```python
from build123d import *

# Parameters (mm, degrees)
SKETCH1_R           = 4
BOSS_EXTRUDE1_DEPTH = 4
SKETCH4_R           = 7
BOSS_EXTRUDE2_DEPTH = 5
SKETCH2_R           = 4.5
SKETCH3_R           = 4


with BuildPart() as part:
    # Sketch1 → Boss-Extrude1 (new body)
    with BuildSketch(Plane(origin=(0, 0, 0), x_dir=(1, 0, 0), z_dir=(0, 1, 0))):
        with BuildLine():
            Line((-3, 300), (-3, 6.32455532))
            ThreePointArc((-3, 6.32455532), (0, -7), (3, 6.32455532))
            Line((3, 6.32455532), (3, 300))
            Line((3, 300), (4.701562119, 301.701562119))
            ThreePointArc((4.701562119, 301.701562119), (4.924825408, 300.863767737), (5, 300))
            Line((5, 300), (10, 300))
            ThreePointArc((10, 300), (0, 310), (-10, 300))
            Line((-10, 300), (-5, 300))
            ThreePointArc((-5, 300), (-4.924825408, 300.863767737), (-4.701562119, 301.701562119))
            Line((-4.701562119, 301.701562119), (-3, 300))
        make_face()
        with Locations(Location((0, 0, 0), (0, 0, 270))):
            Circle(SKETCH1_R, mode=Mode.SUBTRACT)
    extrude(amount=BOSS_EXTRUDE1_DEPTH)

    # Sketch4 → Boss-Extrude2 (add)
    with BuildSketch(Plane(origin=(0, 4, 0), x_dir=(1, 0, 0), z_dir=(0, 1, 0))):
        with Locations(Location((0, 0, 0), (0, 0, 64.623066475))):
            Circle(SKETCH4_R)
    extrude(amount=BOSS_EXTRUDE2_DEPTH)

    # Sketch2 → Cut-Loft1 section 0
    with BuildSketch(Plane(origin=(0, 9, 0), x_dir=(1, 0, 0), z_dir=(0, 1, 0))):
        Circle(SKETCH2_R)
    # Sketch3 → Cut-Loft1 section 1
    with BuildSketch(Plane(origin=(0, 4, 0), x_dir=(1, 0, 0), z_dir=(0, 1, 0))):
        Circle(SKETCH3_R)
    loft(mode=Mode.SUBTRACT)


solid = part.part
```
Work out the finished part from the listing and answer in its coordinate system (mm). A direction names the side the tool comes from. Round coordinates to 2 decimals unless told otherwise and drop trailing zeros. Loops run counter-clockwise (first coordinate to the right, second up) from the corner with the lowest first, then second, coordinate; pieces in that order, holes last. Notation, with made-up numbers: M -34.5,11.25 L 4.5,11.25 A6 cw 4.5,20.25 Z; hole C 36.25,2 d7. An arc over 180 degrees is marked long. One line per question, with ' | ' between items.
Q1. Consider line 1 along X through (y, z) = (2.75, 0); line 2 along Z through (x, y) = (-3.5, 3.25); line 3 along X through (y, z) = (1, -33). Determine where each line is inside the solid, lowest interval first. Write a range as from..to.
Conclusion:
line 1: x = -7..-4, 4..7 | line 2: z = -309.37..-300.5, -6.06..-1.94, 1.94..6.06 | line 3: x = -3..3
Q2. Find section C-C, the plane z = -49.5. Give the vertices of the cut face in (x, y), then the cut area to 3 significant figures.
Conclusion:
outline: M -3,0 L 3,0 L 3,4 L -3,4 Z | area: 24.0 mm2
Q3. Find section A-A, the plane y = 2. Give the vertices of the cut face in (x, z).
Conclusion:
outline: M -10,-300 A10 ccw 10,-300 L 5,-300 A5 cw 4.7,-301.7 L 3,-300 L 3,-6.32 A7 ccw long -3,-6.32 L -3,-300 L -4.7,-301.7 A5 cw -5,-300 Z; hole C 0,0 d8
Q4. Each of these flat-tipped pins is pushed along its axis until it touches: pin 1 Ø10 at (x, z) = (-3.5, -170.5) entering from +Y; pin 2 Ø1.5 at (x, y) = (-2, 4.5) entering from -Z; pin 3 Ø1 at (x, y) = (4, 8) entering from +Z. Where does it stop, or does it pass through?
Conclusion:
pin 1: stops at y = 4 | pin 2: stops at z = -309.9 | pin 3: stops at z = 6.06
Q5. Find section B-B, the plane x = 0. Give the vertices of the cut face in (y, z).
Conclusion:
outline: M 0,-310 L 4,-310 L 4,-7 L 9,-7 L 9,-4.5 L 4,-4 L 0,-4 Z; M 0,4 L 4,4 L 9,4.5 L 9,7 L 0,7 Z
Q6. A tool of negligible diameter and unlimited length cuts with its end or side. For faces 4 (the flat face through (0, 0, -164)), 5 (the flat face through (0, 4, -170)), from which of +Z, -Z, +X, -X, +Y, -Y can it reach the whole face along a straight path? Write none if from no direction.
Conclusion:
face 4: +Z, -Z, +X, -X, -Y | face 5: -Z, +X, -X, +Y
Q7. The mould has two halves that part along Z. Classify faces 1 (the cylindrical face through (0, 2, -310)), 2 (the conical face through (-0.91, 5.91, 4.09)), 3 (the flat face through (5, 9, 1)): +Z half, -Z half, draft (parallel to the pull), parting line (faces both ways), or undercut.
Conclusion:
face 1: -Z half | face 2: undercut | face 3: draft
